Read the model definition and answer for the solid it produces. Units are mm, in the model's axes. A direction names the side the tool comes from. Coordinates: 2 decimals unless noted, no trailing zeros. Order: outer loops, then holes, each group sorted by start corner. A loop starts at its lowest first (then second) coordinate and runs counter-clockwise, first axis right, second up. Notation, with made-up numbers: (-27, 2) -> (28, 2) arc R25 cw to (28, 19) -> close; hole circle Ø4 at (11, 3.5). An arc over 180 degrees is marked (long way). Answer as a JSON object with one key per item and string values. Group by question number.
1) A tool of negligible diameter and unlimited length cuts with its end or side. For faces 1 (the flat face through (7.396, 6.018, -4.191)), 2 (the flat face through (0, 6, -8.5)), 3 (the flat face through (-7.327, 6.018, -4.309)), 4 (the cylindrical face through (-6, 2, 0)), from which of +Z, -Z, +X, -X, +Y, -Y can it reach the whole face along a straight path? Write none if from no direction.
2) Section A-A on x = 0 is taken. Determine the outline of the cut face in (y, z), and give its area (3 significant figures).
3) Given pin 1 (6 mm diameter, centred on x = -1.5, z = -1.5, fed in from -Y); pin 2 (4 mm diameter, centred on y = 32.5, z = -4.5, fed in from -X); pin 3 (1.5 mm diameter, centred on x = -3.5, y = 31.5, fed in from +Z); pin 4 (4 mm diameter, centred on x = 9, y = 18.5, fed in from +Z), each flat-ended and moving along its own axis, determine where each tip first touches the part or whether it passes through.
4) Consider L1, parallel to X at y = 29, z = 0; L2, parallel to Z at x = 0, y = 2.5; L3, parallel to Z at x = 0, y = 15. Determine where each line is inside the solid, lowest interval first.
5) Section C-C on y = 5 is taken. Determine the outline of the cut face in (x, z).
6) Section B-B on z = -1.25 is taken. Determine the outline of the cut face in (x, y).
7) Determine the mould class of faces 5 (the flat face through (0, 23, 2)), 6 (the cylindrical face through (3.434, 2.958, 1.081)), 7 (the cylindrical face through (11.923, 23.583, -3.755)), 8 (the flat face through (7.327, 6.018, 4.309)) for opening direction Z: released by +Z, released by -Z, zero draft, split by the parting line, or undercut.
8) Section D-D on z = 3 is taken. Determine the outline of the cut face in (x, y), and give its area (3 significant figures).
from build123d import *

# Parameters (mm, degrees)
SKETCH1_R           = 6
BOSS_EXTRUDE1_DEPTH = 3.8
BOSS_EXTRUDE2_DEPTH = 4.5
SKETCH3_R           = 12.5
BOSS_EXTRUDE3_DEPTH = 4
SKETCH4_R           = 12.5
BOSS_EXTRUDE4_DEPTH = 27
CUT_EXTRUDE1_DEPTH  = 40.3
SKETCH6_R           = 3.6
CUT_EXTRUDE2_DEPTH  = 6


with BuildPart() as part:
    # Sketch1 → Boss-Extrude1 (new body)
    with BuildSketch(Plane(origin=(0, 0, 0), x_dir=(1, 0, 0), z_dir=(0, 1, 0))):
        Circle(SKETCH1_R)
    extrude(amount=BOSS_EXTRUDE1_DEPTH)

    # Sketch2 → Boss-Extrude2 (add)
    with BuildSketch(Plane(origin=(0, 3.8, 0), x_dir=(1, 0, 0), z_dir=(0, 1, 0))):
        Polygon((9.814954576, 0), (4.907477288, 8.5), (-4.907477288, 8.5), (-9.814954576, 0), (-4.907477288, -8.5), (4.907477288, -8.5), align=None)
    extrude(amount=BOSS_EXTRUDE2_DEPTH)

    # Sketch3 → Boss-Extrude3 (add)
    with BuildSketch(Plane(origin=(0, 8.3, 0), x_dir=(1, 0, 0), z_dir=(0, 1, 0))):
        Circle(SKETCH3_R)
    extrude(amount=BOSS_EXTRUDE3_DEPTH)

    # Sketch4 → Boss-Extrude4 (add)
    with BuildSketch(Plane(origin=(0, 12.3, 0), x_dir=(1, 0, 0), z_dir=(0, 1, 0))):
        Circle(SKETCH4_R)
    extrude(amount=BOSS_EXTRUDE4_DEPTH)

    # Sketch5 → Cut-Extrude1 (cut, through all)
    with BuildSketch(Plane(origin=(0, 39.3, 0), x_dir=(1, 0, 0), z_dir=(0, 1, 0))):
        with BuildLine():
            ThreePointArc((3, 0), (-1.070466269, 2.802517077), (-2.236067977, -2))
            Line((-2.236067977, -2), (2.236067977, -2))
            ThreePointArc((2.236067977, -2), (2.802517077, -1.070466269), (3, 0))
        make_face()
    extrude(amount=-CUT_EXTRUDE1_DEPTH, mode=Mode.SUBTRACT)

    # Sketch6 → Cut-Extrude2 (cut)
    with BuildSketch(Plane.XZ):
        Circle(SKETCH6_R)
    extrude(amount=-CUT_EXTRUDE2_DEPTH, mode=Mode.SUBTRACT)


solid = part.part
Worked answers:
{
 "1": {"face 1": "-Z, +X, -Y", "face 2": "-Z, +X, -X, -Y", "face 3": "-Z, -X, -Y", "face 4": "-Y"},
 "2": {"outline": "(0, -6) -> (3.8, -6) -> (3.8, -8.5) -> (8.3, -8.5) -> (8.3, -12.5) -> (39.3, -12.5) -> (39.3, -3) -> (6, -3) -> (6, -3.6) -> (0, -3.6) -> close; (0, 3.6) -> (6, 3.6) -> (6, 2) -> (39.3, 2) -> (39.3, 12.5) -> (8.3, 12.5) -> (8.3, 8.5) -> (3.8, 8.5) -> (3.8, 6) -> (0, 6) -> close", "area": "687 mm²"},
 "3": {"pin 1": "stops at y = 0", "pin 2": "stops at x = -12.25", "pin 3": "stops at z = 12.19", "pin 4": "stops at z = 10.36"},
 "4": {"L1": "x = -12.5 to -3, 3 to 12.5", "L2": "z = -6 to -3.6, 3.6 to 6", "L3": "z = -12.5 to -3, 2 to 12.5"},
 "5": {"outline": "(-9.81, 0) -> (-4.91, -8.5) -> (4.91, -8.5) -> (9.81, 0) -> (4.91, 8.5) -> (-4.91, 8.5) -> close; hole circle Ø7.2 at (0, 0)"},
 "6": {"outline": "(-12.44, 8.3) -> (-9.09, 8.3) -> (-9.09, 3.8) -> (-5.87, 3.8) -> (-5.87, 0) -> (-3.38, 0) -> (-3.38, 6) -> (-2.73, 6) -> (-2.73, 39.3) -> (-12.44, 39.3) -> close; (2.73, 6) -> (3.38, 6) -> (3.38, 0) -> (5.87, 0) -> (5.87, 3.8) -> (9.09, 3.8) -> (9.09, 8.3) -> (12.44, 8.3) -> (12.44, 39.3) -> (2.73, 39.3) -> close"},
 "7": {"face 5": "undercut", "face 6": "undercut", "face 7": "split by the parting line", "face 8": "released by +Z"},
 "8": {"outline": "(-12.13, 8.3) -> (-8.08, 8.3) -> (-8.08, 3.8) -> (-5.2, 3.8) -> (-5.2, 0) -> (-1.99, 0) -> (-1.99, 6) -> (1.99, 6) -> (1.99, 0) -> (5.2, 0) -> (5.2, 3.8) -> (8.08, 3.8) -> (8.08, 8.3) -> (12.13, 8.3) -> (12.13, 39.3) -> (-12.13, 39.3) -> close", "area": "841 mm²"}
}
